Read the model definition and answer for the solid it produces. Units are mm, in the model's axes. Face numbers are marked on the shaded views. A direction names the side the tool comes from. Round coordinates to 2 decimals unless told otherwise and drop trailing zeros. Loops run counter-clockwise (first coordinate to the right, second up) from the corner with the lowest first, then second, coordinate; pieces in that order, holes last. Notation, with made-up numbers: M 74.5,85.25 L 92.5,85.25 A20 ccw 92.5,107.25 Z; hole C 55,-5.75 d2. An arc over 180 degrees is marked long. Write each question's results on one line, items separated by ' | '.
from build123d import *

# Parameters (mm, degrees)
F3_DEPTH = 8.001


with BuildPart() as f1:
    # F0 (on Front) → F1 (revolve)
    with BuildSketch(Plane.XZ):
        Polygon((0, 2), (0, 0), (15.4, 0), (15.4, 2), (14.6, 2), align=None)
        Polygon((15.4, 2), (15.4, 0), (17.4, 2), (15.6, 2), align=None)
        Polygon((14.6, 2), (15.4, 2), (15.6, 2), (15.6, 6), (15.6, 10), (14.6, 10), align=None)
        Polygon((15.6, 10), (15.6, 6), (16.6, 8), align=None)
    revolve(axis=Axis((0, 0, 1), (0, 0, 1)))

    # F2 (on face) → F3 (cut, through all)
    with BuildSketch(Plane.XY.offset(2)):
        with BuildLine():
            Line((0, 19), (0, 0))
            Line((0, 0), (16.454483, 9.5))
            ThreePointArc((16.454483, 9.5), (9.5, 16.454483), (0, 19))
        make_face()
        with BuildLine():
            Line((-16.454483, -9.5), (0, 0))
            Line((0, 0), (-16.454483, 9.5))
            ThreePointArc((-16.454483, 9.5), (-19, 0), (-16.454483, -9.5))
        make_face()
        with BuildLine():
            Line((16.454483, -9.5), (0, 0))
            Line((0, 0), (0, -19))
            ThreePointArc((0, -19), (9.5, -16.454483), (16.454483, -9.5))
        make_face()
    extrude(amount=F3_DEPTH, mode=Mode.SUBTRACT)


solid = f1.part
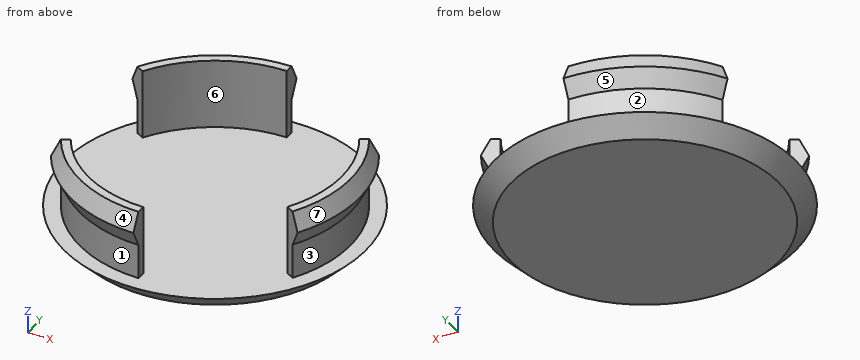
Item 1: The part is cut by section A-A (z = 4). Determine the outline of the cut face in (x, y).
Outcome:
outline: M -13.51,-7.8 A15.6 ccw 0,-15.6 L 0,-14.6 A14.6 cw -12.64,-7.3 Z; M -13.51,7.8 L -12.64,7.3 A14.6 cw 0,14.6 L 0,15.6 A15.6 ccw Z; M 12.64,-7.3 L 13.51,-7.8 A15.6 ccw 13.51,7.8 L 12.64,7.3 A14.6 cw Z
Item 2: The part is cut by section C-C (z = 6.5). State how many separate pieces and enclosed holes the cut face has, plus the area to 3 significant figures.
Outcome:
separate pieces: 3 | enclosed holes: 0 | area: 59.8 mm2
Item 3: Straight lines are drawn through the part: line 1 (Z direction, x = -13.5, y = 3.5); line 2 (Y direction, x = -5.5, z = 6.75); line 3 (X direction, y = -9, z = 1.75). For each, find the intervals that lie inside material, in ascending order.
Outcome:
line 1: z = 0 to 2 | line 2: y = -15 to -13.52, 13.52 to 15 | line 3: x = -14.6 to 14.6
Item 4: Flat-ended cylindrical pins translate along their axes: pin 1 (2 mm diameter, centred on y = 15, z = 7, fed in from +X); pin 2 (1.5 mm diameter, centred on x = -13, z = 4.5, fed in from +Y); pin 3 (1 mm diameter, centred on y = 11, z = 8, fed in from -X). Find the tip coordinate at first contact, or state that the pin passes through.
Outcome:
pin 1: stops at x = 0 | pin 2: stops at y = 9.66 | pin 3: stops at x = -12.86
Item 5: For the marked faces 1, 2, 3 and 4, determine the directions among +Z, -Z, +X, -X, +Y, -Y from which every point of the face is accessible in a straight line to the end or side of a thin tool.
Outcome:
face 1: -X, -Y | face 2: -X, +Y | face 3: +X | face 4: +Z, -X, -Y
Item 6: The mould has two halves that part along Y. Classify the marked faces 5, 6 and 7: pulls with the +Y half, pulls with the -Y half, needs draft (parallel to the pull), parting line crosses it, or undercut.
Outcome:
face 5: pulls with the +Y half | face 6: undercut | face 7: parting line crosses it
Item 7: The part is cut by section B-B (y = 0). Determine the outline of the cut face in (x, z).
Outcome:
outline: M -17.4,2 L -15.4,0 L 15.4,0 L 17.4,2 L 15.6,2 L 15.6,6 L 16.6,8 L 15.6,10 L 14.6,10 L 14.6,2 Z
